Work out the finished part from the listing and answer in its coordinate system (mm). A direction names the side the tool comes from. Coordinates: 2 decimals unless noted, no trailing zeros. Loops run counter-clockwise (first coordinate to the right, second up) from the corner with the lowest first, then second, coordinate; pieces in that order, holes last. Notation, with made-up numbers: (65.5, 23.25) -> (83.5, 23.25) arc R23 ccw to (83.5, 34.25) -> close; hole circle Ø10 at (49.25, -23.75). An arc over 180 degrees is marked (long way). Answer as CSV lines item,"result".
Autodesk Inventor part; units mm, degrees
ref_plane "dia1_XY" through (0, 3.175, 0) normal (1, 0, 0) x (0, 0, -1)
ref_plane "dia1_YZ" through (0, 3.175, 0) normal (0, 0, -1) x (0, 1, 0)
ref_plane "dia1_ZX" through (0, 3.175, 0) normal (0, 1, 0) x (1, 0, 0)
sketch "Sketch_1" plane through (0, 0, 0) normal (0, 0, 1) x (1, 0, 0)
  line L0 (73.152, 0) -> (0, 0)
  line L1 (0, 0) -> (0, 3.175)
  line L2 (0, 3.175) -> (53.1876, 3.175)
  line L3 (53.1876, 3.175) -> (53.1876, 9.6203)
  line L4 (53.1876, 9.6203) -> (73.152, 9.6203)
  line L5 (73.152, 9.6203) -> (73.152, 0)
  line L6 (73.152, 0) -> (0, 0)
revolve "Revolution1" add sketch "Sketch_1" angle 360 about axis through (73.152, 0, 0) along (1, 0, 0)
sketch "Sketch_3" plane through (0, 0, 0) normal (0, 0, 1) x (1, 0, 0)
  line L0 (0, 0) -> (-12.7, 0)
  line L1 (-12.7, 0) -> (-12.7, 2.634)
  line L2 (-12.7, 2.634) -> (-12.159, 3.175)
  line L3 (-12.159, 3.175) -> (0, 3.175)
  line L4 (0, 3.175) -> (0, 0)
  line L5 (0, 0) -> (-12.7, 0)
revolve "Revolution2" add sketch "Sketch_3" angle 360 about axis through (0, 0, 0) along (1, 0, 0)
thread "Thread1"
sketch "Sketch_30" plane through (0, 0, 0) normal (0, 0, 1) x (1, 0, 0)
  line L0 (0, 0) -> (-0.254, 0)
  line L1 (-0.254, 2.921) -> (0, 2.921)
  line L2 (0, 2.921) -> (0, 3.429)
  line L3 (0, 3.429) -> (-0.254, 3.429)
  line L4 (-0.254, 3.429) -> (-0.254, 2.921)
revolve "Revolution3" cut sketch "Sketch_30" angle 360 about axis through (0, 0, 0) along (1, 0, 0)
ref_plane "dia1_XY" through (0, 3.175, 0) normal (1, 0, 0) x (0, 0, -1)
ref_plane "dia1_YZ" through (0, 3.175, 0) normal (0, 0, -1) x (0, 1, 0)
ref_plane "dia1_ZX" through (0, 3.175, 0) normal (0, 1, 0) x (1, 0, 0)
ref_plane "dia12_XY" through (0, 0, 10.9537) normal (1, 0, 0) x (0, 0, -1)
ref_plane "dia12_YZ" through (0, 0, 10.9537) normal (0, 0, -1) x (0, 1, 0)
ref_plane "dia12_ZX" through (0, 0, 10.9537) normal (0, 1, 0) x (1, 0, 0)
ref_plane "dia1r_XY" through (0, 0, 10.2235) normal (1, 0, 0) x (0, 0, -1)
ref_plane "dia1r_YZ" through (0, 0, 10.2235) normal (0, 0, -1) x (0, 1, 0)
ref_plane "dia1r_ZX" through (0, 0, 10.2235) normal (0, 1, 0) x (1, 0, 0)
ref_plane "dia2_XY" through (0, -3.175, 0) normal (1, 0, 0) x (0, 0, -1)
ref_plane "dia2_YZ" through (0, -3.175, 0) normal (0, 0, -1) x (0, 1, 0)
ref_plane "dia2_ZX" through (0, -3.175, 0) normal (0, 1, 0) x (1, 0, 0)
ref_plane "dia22_XY" through (0, 0, -10.9537) normal (1, 0, 0) x (0, 0, -1)
ref_plane "dia22_YZ" through (0, 0, -10.9537) normal (0, 0, -1) x (0, 1, 0)
ref_plane "dia22_ZX" through (0, 0, -10.9537) normal (0, 1, 0) x (1, 0, 0)
ref_plane "dia2r_XY" through (0, 0, -10.2235) normal (1, 0, 0) x (0, 0, -1)
ref_plane "dia2r_YZ" through (0, 0, -10.2235) normal (0, 0, -1) x (0, 1, 0)
ref_plane "dia2r_ZX" through (0, 0, -10.2235) normal (0, 1, 0) x (1, 0, 0)
ref_plane "rl1_XY" through (-12.7, 0, 0) normal (1, 0, 0) x (0, 0, -1)
ref_plane "rl1_YZ" through (-12.7, 0, 0) normal (0, 0, -1) x (0, 1, 0)
ref_plane "rl1_ZX" through (-12.7, 0, 0) normal (0, 1, 0) x (1, 0, 0)
ref_plane "rl2_XY" through (0, 0, 0) normal (1, 0, 0) x (0, 0, -1)
ref_plane "rl2_YZ" through (0, 0, 0) normal (0, 0, -1) x (0, 1, 0)
ref_plane "rl2_ZX" through (0, 0, 0) normal (0, 1, 0) x (1, 0, 0)
ref_plane "rod_cp_XY" through (0, 0, 0) normal (1, 0, 0) x (0, 0, -1)
ref_plane "rod_cp_YZ" through (0, 0, 0) normal (0, 0, -1) x (0, 1, 0)
ref_plane "rod_cp_ZX" through (0, 0, 0) normal (0, 1, 0) x (1, 0, 0)
ref_plane "stroke1_XY" through (0, 0, 0) normal (1, 0, 0) x (0, 0, -1)
ref_plane "stroke1_YZ" through (0, 0, 0) normal (0, 0, -1) x (0, 1, 0)
ref_plane "stroke1_ZX" through (0, 0, 0) normal (0, 1, 0) x (1, 0, 0)
ref_plane "thd1_XY" through (-12.7, 3.175, 0) normal (1, 0, 0) x (0, 0, -1)
ref_plane "thd1_YZ" through (-12.7, 3.175, 0) normal (0, 0, -1) x (0, 1, 0)
ref_plane "thd1_ZX" through (-12.7, 3.175, 0) normal (0, 1, 0) x (1, 0, 0)
ref_plane "thd2_XY" through (-12.7, -3.175, 0) normal (1, 0, 0) x (0, 0, -1)
ref_plane "thd2_YZ" through (-12.7, -3.175, 0) normal (0, 0, -1) x (0, 1, 0)
ref_plane "thd2_ZX" through (-12.7, -3.175, 0) normal (0, 1, 0) x (1, 0, 0)
ref_plane "to_rod_clevis_XY" through (-16.764, 0, 0) normal (1, 0, 0) x (0, 0, -1)
ref_plane "to_rod_clevis_YZ" through (-16.764, 0, 0) normal (0, 0, -1) x (0, 1, 0)
ref_plane "to_rod_clevis_ZX" through (-16.764, 0, 0) normal (0, 1, 0) x (1, 0, 0)
properties part number "C-040.5-RP0000_rod"
(1) Consider line 1 along X through (y, z) = (4.75, -2.5); line 2 along Z through (x, y) = (-6, 0) (3 decimals); line 3 along Y through (x, z) = (26, -0.25). Determine where each line is inside the solid, lowest interval first.
Computed values:
line 1,"53.19 to 73.15"
line 2,"-3.175 to 3.175"
line 3,"-3.17 to 3.17"
(2) A cutting plane is placed at C-C, the plane x = 35. Write down the section's boundary in (y, z) (3 decimals), and give its area (3 significant figures).
Computed values:
outline,"circle Ø6.35 at (0, 0)"
area,"31.7 mm2"
(3) A cutting plane is placed at D-D, the plane y = 5.25. Write down the section's boundary in (x, z), and give its area (3 significant figures).
Computed values:
outline,"(53.19, -8.06) -> (73.15, -8.06) -> (73.15, 8.06) -> (53.19, 8.06) -> close"
area,"322 mm2"
(4) A flat-ended cylindrical pin translates along its axis: pin 1 Ø3 at (x, y) = (22.5, -5) entering from -Z. Find the tip coordinate at first contact, or state that the pin passes through.
Computed values:
pin 1,"through"
(5) Which of the six approach directions +Z, -Z, +X, -X, +Y, -Y give full straight-line access (tool end or side, diameter ignored) to faces 1 (the face through (26.97, -0.69, -3.1)), 2 (the face through (63.31, -2.09, -9.39))?
Computed values:
face 1,"-X"
face 2,"+X, -X"
(6) A cutting plane is placed at A-A, the plane y = 0. Write down the section's boundary in (x, z) (3 decimals), and give its area (3 significant figures).
Computed values:
outline,"(-12.7, -2.634) -> (-12.159, -3.175) -> (-0.254, -3.175) -> (-0.254, -2.921) -> (0, -2.921) -> (0, -3.175) -> (53.188, -3.175) -> (53.188, -9.62) -> (73.152, -9.62) -> (73.152, 9.62) -> (53.188, 9.62) -> (53.188, 3.175) -> (0, 3.175) -> (0, 2.921) -> (-0.254, 2.921) -> (-0.254, 3.175) -> (-12.159, 3.175) -> (-12.7, 2.634) -> close"
area,"802 mm2"
